The figure shows three views and two pictorial views of one solid part (mm, origin at its lowest corner). Answer the questions. A direction names the side the tool comes from. Round coordinates to 2 decimals unless told otherwise and drop trailing zeros. Order: outer loops, then holes, each group sorted by start corner. A loop starts at its lowest first (then second) coordinate and runs counter-clockwise, first axis right, second up. Notation, with made-up numbers: (40, 77) - (66, 77) arc R22 ccw to (66, 100) - close; hole circle Ø1 at (34.25, -19). An arc over 180 degrees is marked (long way). Use CSV: the item, a comma, the result in double quotes.
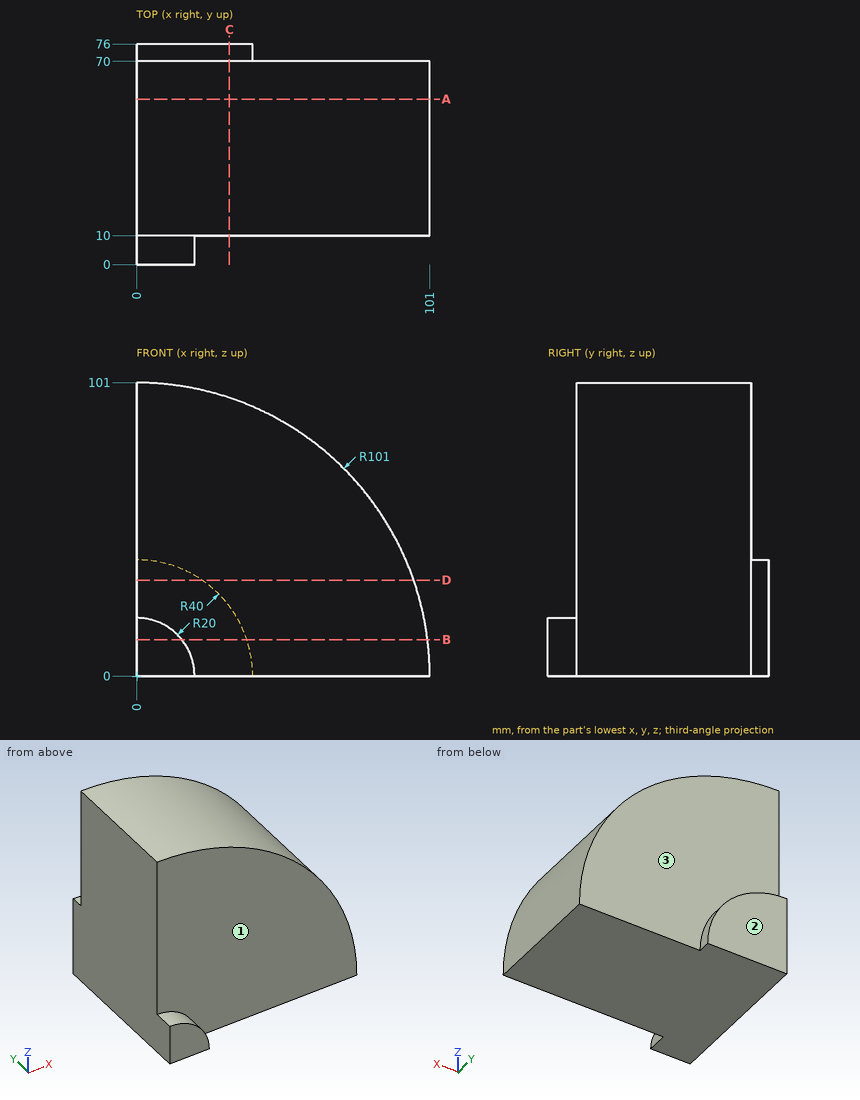
(1) Find section B-B (z = 12.5). Determine the outline of the cut face in (x, y).
Findings below:
outline,"(0, 0) - (15.61, 0) - (15.61, 10) - (100.22, 10) - (100.22, 70) - (38, 70) - (38, 76) - (0, 76) - close"
(2) Each of these flat-tipped pins is pushed along its axis until it touches: pin 1 (5 mm diameter, centred on y = 62, z = 60, fed in from +X); pin 2 (1 mm diameter, centred on x = 44.5, z = 26, fed in from +Y); pin 3 (2 mm diameter, centred on y = 8.5, z = 70.5, fed in from -X). Where does it stop, or does it pass through?
Findings below:
pin 1,"stops at x = 83.03"
pin 2,"stops at y = 70"
pin 3,"passes through"
(3) Find section C-C (x = 32). Determine the outline of the cut face in (y, z), and give its area (3 significant figures).
Findings below:
outline,"(10, 0) - (76, 0) - (76, 24) - (70, 24) - (70, 95.8) - (10, 95.8) - close"
area,"5,890 mm²"
(4) For the marked faces 1, 2 and 3, determine the directions among +Z, -Z, +X, -X, +Y, -Y from which every point of the face is accessible in a straight line to the end or side of a thin tool.
Findings below:
face 1,"+Z, +X, -Y"
face 2,"+Z, -Z, +X, -X, +Y"
face 3,"+Z, +X, +Y"
(5) Find section D-D (z = 33). Determine the outline of the cut face in (x, y).
Findings below:
outline,"(0, 10) - (95.46, 10) - (95.46, 70) - (22.61, 70) - (22.61, 76) - (0, 76) - close"
(6) Find section A-A (y = 57). Determine the outline of the cut face in (x, z), and give its area (3 significant figures).
Findings below:
outline,"(0, 0) - (101, 0) arc R101 ccw to (0, 101) - close"
area,"8,010 mm²"
(7) Find the intervals of material crossed by L1, parallel to Y at x = 9, z = 50.5; L2, parallel to Y at x = 23, z = 29; L3, parallel to X at y = 22, z = 37, in increasing order. Write a range as from..to.
Findings below:
L1,"y = 10..70"
L2,"y = 10..76"
L3,"x = 0..93.98"
